Check sheet for the modelled part. Datum: model origin and axes. Units: mm. Face numbers are marked on the shaded views. Round coordinates to 2 decimals unless told otherwise and drop trailing zeros. Write each loop counter-clockwise with the first axis right and the second up, starting at its lowest first coordinate (ties: lowest second). Pieces come first, ordered by that corner, then holes. Notation, with made-up numbers: M 58.25,51.5 L 116.25,51.5 A23 cw 116.25,61.5 Z; hole C 76.5,-25 d5. An arc over 180 degrees is marked long. Answer in a Markdown table with one row per item.
```python
from build123d import *


with BuildPart() as f1:
    # F0 (on Front) → F1 (revolve)
    with BuildSketch(Plane.XZ):
        with BuildLine():
            Line((0, 6.35), (0, 0))
            Line((0, 0), (50.8, 0))
            Line((50.8, 0), (50.8, 101.6))
            Line((50.8, 101.6), (0, 29.050081))
            Line((0, 29.050081), (0, 21.717098))
            ThreePointArc((0, 21.717098), (2.920268, 23.11225), (5.201615, 25.407871))
            Line((5.201615, 25.407871), (44.45, 81.460373))
            Line((44.45, 81.460373), (44.45, 6.35))
            Line((44.45, 6.35), (0, 6.35))
        make_face()
    revolve(axis=Axis((0, 0, 14.525041), (0, 0, -1)))


solid = f1.part
```
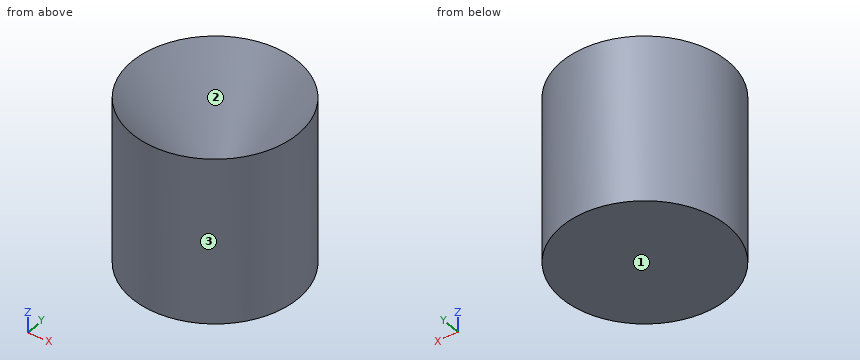
1. Draft check along X on the marked faces 1, 2 and 3. Enter one of: +X half, -X half, draft (parallel to the pull), parting line (faces both ways), or undercut.
Found:
| item | result |
|---|---|
| face 1 | draft |
| face 2 | undercut |
| face 3 | parting line |
2. Section check C-C, the plane z = 35. Record the cut outline in (x, y).
Found:
| item | result |
|---|---|
| outline | C 0,0 d101.6; C 0,0 d23.84; hole C 0,0 d88.9; hole C 0,0 d8.33 |
3. Section check A-A, the plane z = 71.5. Record the cut outline in (x, y), and give its area (3 significant figures).
Found:
| item | result |
|---|---|
| outline | C 0,0 d101.6; C 0,0 d74.95; hole C 0,0 d88.9; hole C 0,0 d59.45 |
| area | 3,540 mm2 |
4. Scan lines: L1, parallel to Y at x = 0, z = 30.5; L2, parallel to Y at x = 6, z = 56; L3, parallel to X at y = 0, z = 54. Record each from-to range of solid material in increasing order.
Found:
| item | result |
|---|---|
| L1 | y = -50.8 to -44.45, -8.77 to -1.02, 1.02 to 8.77, 44.45 to 50.8 |
| L2 | y = -50.44 to -44.04, -25.94 to -17.89, 17.89 to 25.94, 44.04 to 50.44 |
| L3 | x = -50.8 to -44.45, -25.22 to -17.47, 17.47 to 25.22, 44.45 to 50.8 |
5. Go/stop test with flat-tipped pins: pin 1 (6 mm diameter, centred on y = 16, z = 43.5, fed in from +X); pin 2 (1.5 mm diameter, centred on x = -14.5, z = 29.5, fed in from -Y); pin 3 (12 mm diameter, centred on x = 6, z = 80.5, fed in from +Y). Record where each tip stops, or that it passes through.
Found:
| item | result |
|---|---|
| pin 1 | stops at x = 49.11 |
| pin 2 | stops at y = -48.9 |
| pin 3 | stops at y = 50.8 |
6. Section check B-B, the plane z = 9. Record the cut outline in (x, y).
Found:
| item | result |
|---|---|
| outline | C 0,0 d101.6; hole C 0,0 d88.9 |
